The model under review builds one solid part; all positions refer to its coordinate system, in mm. Face numbers are marked on the shaded views. A direction names the side the tool comes from. Coordinates: 2 decimals unless noted, no trailing zeros. Order: outer loops, then holes, each group sorted by start corner. A loop starts at its lowest first (then second) coordinate and runs counter-clockwise, first axis right, second up. Notation, with made-up numbers: (68.25, 63) -> (83.25, 63) arc R15 cw to (83.25, 81) -> close; hole circle Ø3 at (12, -34.5). An arc over 180 degrees is marked (long way). Use one line per item in the form item = value.
from build123d import *

# Parameters (mm, degrees)
SKETCH1_W           = 20.32
SKETCH1_H           = 10.16
BOSS_EXTRUDE1_DEPTH = 1.27
SKETCH2_W           = 10.16
SKETCH2_H           = 5.08
CUT_EXTRUDE1_DEPTH  = 12.43
SKETCH4_W           = 20.32
SKETCH4_H           = 0.79375
BOSS_EXTRUDE2_DEPTH = 1.27
SKETCH5_W           = 5.08
SKETCH5_H           = 1.27
CUT_EXTRUDE2_DEPTH  = 1.27
FILLET1_R           = 1.27


with BuildPart() as part:
    # Sketch1 → Boss-Extrude1 (new body)
    with BuildSketch(Plane(origin=(0, 0, 0), x_dir=(1, 0, 0), z_dir=(0, 1, 0))):
        Rectangle(SKETCH1_W, SKETCH1_H)
    extrude(amount=BOSS_EXTRUDE1_DEPTH)

    # Sketch2 → Cut-Extrude1 (cut, through all)
    with BuildSketch(Plane(origin=(0, 1.27, 0), x_dir=(1, 0, 0), z_dir=(0, 1, 0))):
        with Locations((0, -2.54)):
            Rectangle(SKETCH2_W, SKETCH2_H)
    extrude(amount=-CUT_EXTRUDE1_DEPTH, mode=Mode.SUBTRACT)

    # Sketch4 → Boss-Extrude2 (add)
    with BuildSketch(Plane(origin=(0, 1.27, 0), x_dir=(1, 0, 0), z_dir=(0, 1, 0))):
        with Locations((0, 4.683125)):
            Rectangle(SKETCH4_W, SKETCH4_H)
    extrude(amount=BOSS_EXTRUDE2_DEPTH)

    # Sketch5 → Cut-Extrude2 (cut)
    with BuildSketch(Plane.XY.offset(5.08)):
        with Locations((7.62, 0.635)):
            Rectangle(SKETCH5_W, SKETCH5_H)
        with Locations((-7.62, 0.635)):
            Rectangle(SKETCH5_W, SKETCH5_H)
    extrude(amount=-CUT_EXTRUDE2_DEPTH, mode=Mode.SUBTRACT)

    # Fillet1
    fillet1_edges = [part.edges().sort_by_distance(p)[0] for p in [
        (10.16, 1.27, -5.08),
        (5.08, 0.635, 0),
        (-5.08, 0.635, 0),
        (-10.16, 1.27, -5.08),
    ]]
    fillet(fillet1_edges, radius=FILLET1_R)


solid = part.part
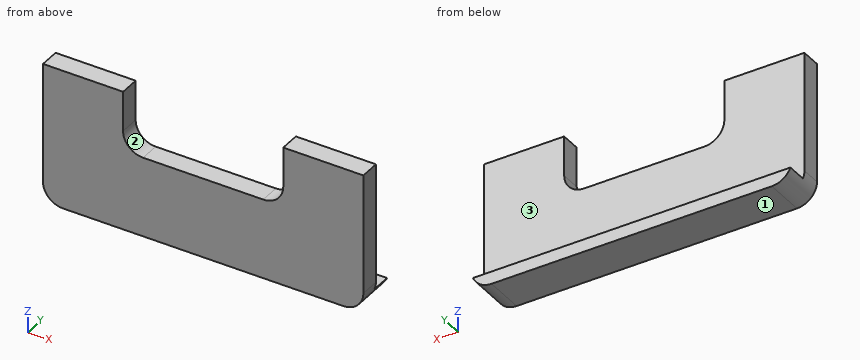
Item 1: We need section D-D (z = -3). Write out the cut boundary in (x, y).
Results found:
outline = (-10.16, 0) -> (10.16, 0) -> (10.16, 1.27) -> (-10.16, 1.27) -> close
Item 2: We need section C-C (x = 0.75). Write out the cut boundary in (y, z), plus the area to 3 significant figures.
Results found:
outline = (0, -5.08) -> (2.54, -5.08) -> (2.54, -4.29) -> (1.27, -4.29) -> (1.27, 0) -> (0, 0) -> close
area = 7.46 mm²
Item 3: Clearance check with flat-ended pins moving along their axes: pin 1 (2 mm diameter, centred on x = 0, z = -2.5, fed in from +Y); pin 2 (1 mm diameter, centred on y = 2, z = -0.5, fed in from -X); pin 3 (1.4 mm diameter, centred on x = 1, y = 1.5, fed in from +Z). State where each tip first meets the part, or that it passes through.
Results found:
pin_1 = 1.27
pin_2 = through
pin_3 = 0
Item 4: Tool access review of the marked faces 1, 2 and 3: name each direction out of +Z, -Z, +X, -X, +Y, -Y from which nothing blocks a thin tool from reaching the whole face with its end or side.
Results found:
face_1 = -Z, +X, -X, +Y, -Y
face_2 = +Z, +Y, -Y
face_3 = +Z, +X, -X, +Y
Item 5: To check wall thickness, follow L1, parallel to Y at x = 4, z = -3.5; L2, parallel to Z at x = -3, y = 0.55; L3, parallel to X at y = 0.55, z = 1.5. State the ranges of each line that lie inside material, in increasing order. Write a range as from..to.
Results found:
L1 = 0..1.27
L2 = -5.08..0
L3 = -10.16..-5.08, 5.08..10.16
Item 6: We need section B-B (y = 0.75). Write out the cut boundary in (x, z).
Results found:
outline = (-10.16, -3.81) arc R1.27 ccw to (-8.89, -5.08) -> (8.89, -5.08) arc R1.27 ccw to (10.16, -3.81) -> (10.16, 3.81) -> (5.08, 3.81) -> (5.08, 1.27) arc R1.27 cw to (3.81, 0) -> (-3.81, 0) arc R1.27 cw to (-5.08, 1.27) -> (-5.08, 3.81) -> (-10.16, 3.81) -> close
Item 7: We need section A-A (z = 1). Write out the cut boundary in (x, y).
Results found:
outline = (-10.16, 0) -> (-5.05, 0) -> (-5.05, 1.27) -> (-10.16, 1.27) -> close; (5.05, 0) -> (10.16, 0) -> (10.16, 1.27) -> (5.05, 1.27) -> close
